Answer from the drawing. Dimensions are ordinates in mm from the lowest x, y and z of the part. A direction names the side the tool comes from. Round coordinates to 2 decimals unless told otherwise and drop trailing zeros. Order: outer loops, then holes, each group sorted by start corner. A loop starts at its lowest first (then second) coordinate and runs counter-clockwise, first axis right, second up. Notation, with made-up numbers: (9, 44) - (47, 44) arc R11 cw to (47, 57) - close; hole circle Ø8 at (-35, 17). An arc over 180 degrees is marked (long way). One line per question, with ' | ' between items. Start each with the question number.
1) Straight lines are drawn through the part: line 1 (X direction, y = 0.5, z = 49.5); line 2 (Z direction, x = 16, y = 2.75) (1 decimal); line 3 (Z direction, x = 26, y = 2) (1 decimal). For each, find the intervals that lie inside material, in ascending order. Write a range as from..to.
2) The mould has two halves that part along Y. Classify the marked faces 3, 4 and 5: pulls with the +Y half, pulls with the -Y half, needs draft (parallel to the pull), parting line crosses it, or undercut.
3) For the marked faces 1 and 2, determine the directions among +Z, -Z, +X, -X, +Y, -Y from which every point of the face is accessible in a straight line to the end or side of a thin tool.
4) The part is cut by section B-B, the plane y = 1.5. Give the vertices of the cut face in (x, z) (1 decimal).
5) The part is cut by section A-A, the plane z = 5. Give the vertices of the cut face in (x, y), plus the area to 3 significant figures.
6) Flat-ended cylindrical pins translate along their axes: pin 1 (3 mm diameter, centred on y = 3.5, z = 23.5, fed in from +X); pin 2 (1.5 mm diameter, centred on x = 20, y = 7, fed in from +Z) (1 decimal); pin 3 (1 mm diameter, centred on x = 25, y = 4, fed in from -Z). Find the tip coordinate at first contact, or state that the pin passes through.
7) The part is cut by section C-C, the plane x = 22.5. Give the vertices of the cut face in (y, z).
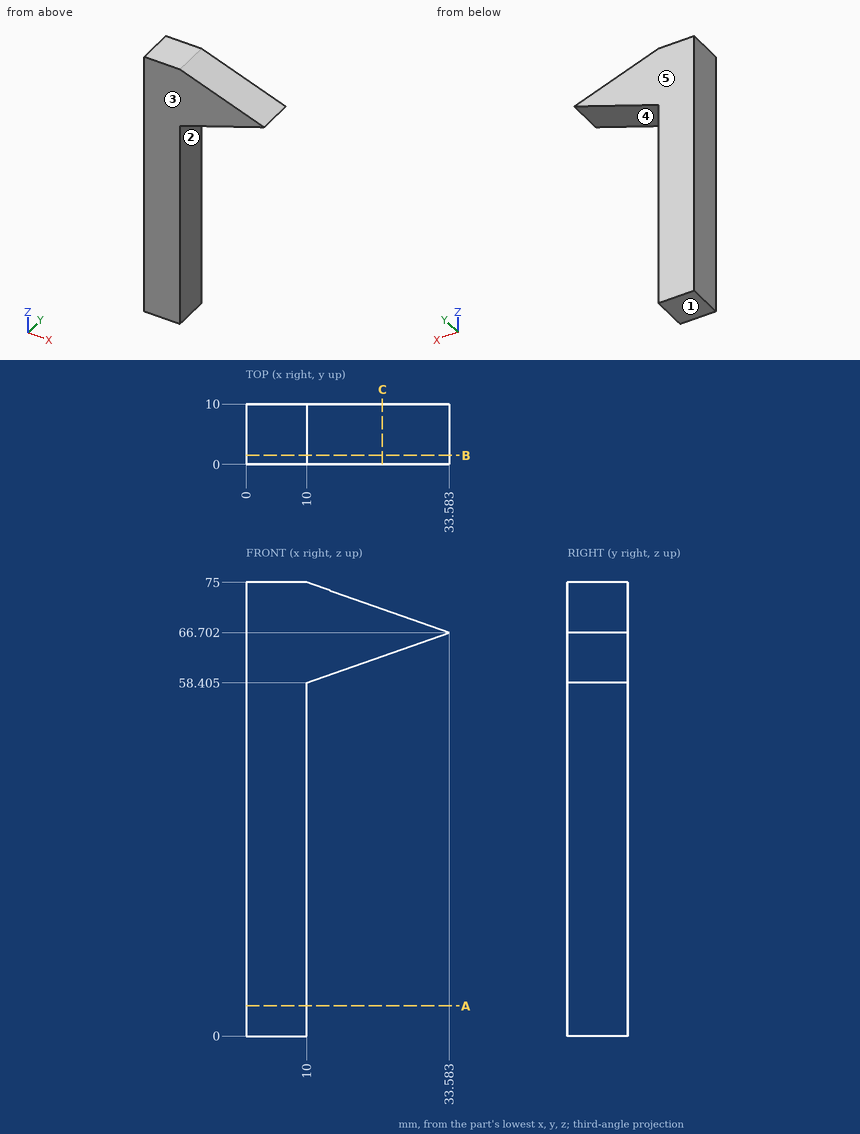
Values:
1) line 1: x = 0..10 | line 2: z = 60.5..72.9 | line 3: z = 64..69.4
2) face 3: pulls with the -Y half | face 4: needs draft | face 5: pulls with the +Y half
3) face 1: -Z, +X, -X, +Y, -Y | face 2: -Z, +X, +Y, -Y
4) outline: (0, 0) - (10, 0) - (10, 58.4) - (33.6, 66.7) - (10, 75) - (0, 75) - close
5) outline: (0, 0) - (10, 0) - (10, 10) - (0, 10) - close | area: 100 mm^2
6) pin 1: stops at x = 10 | pin 2: stops at z = 71.7 | pin 3: stops at z = 63.51
7) outline: (0, 62.8) - (10, 62.8) - (10, 70.6) - (0, 70.6) - close
